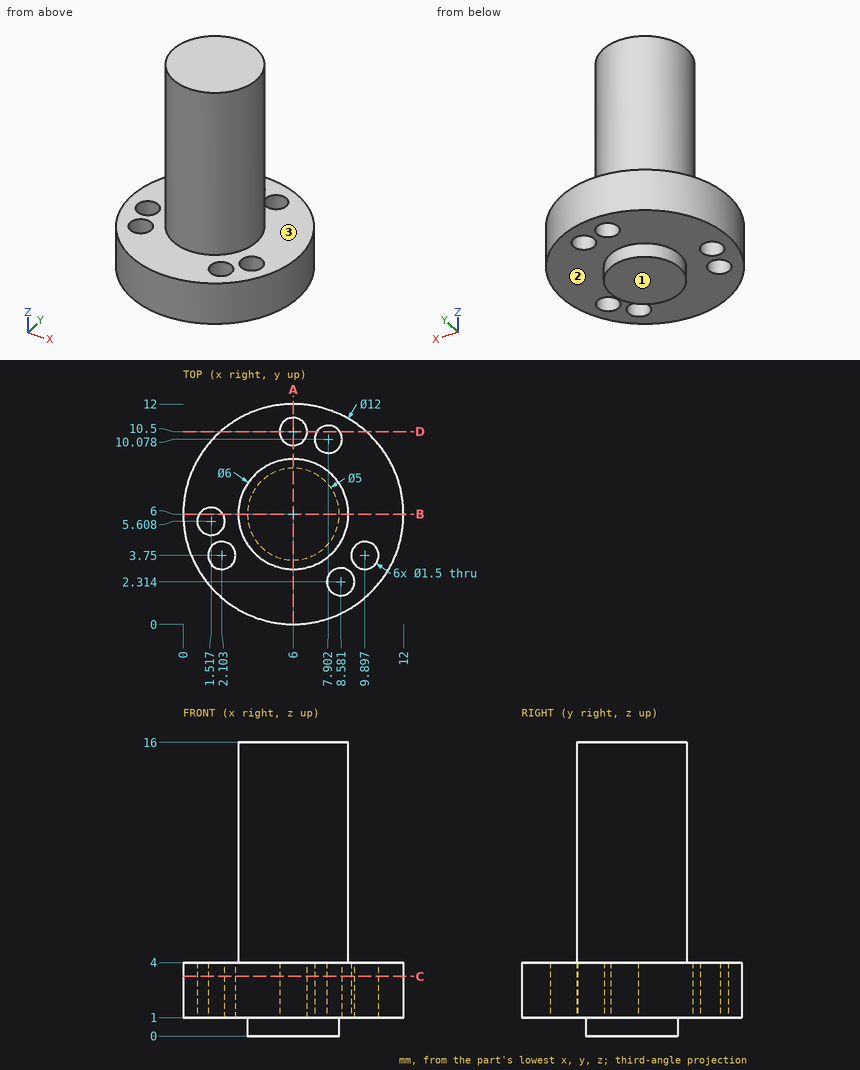
Design review of the part shown in the three views and the two pictorial views. Dimensions are in mm from the part's minimum x, y and z. A direction names the side the tool comes from. Round coordinates to 2 decimals unless told otherwise and drop trailing zeros. Order: outer loops, then holes, each group sorted by start corner. A loop starts at its lowest first (then second) coordinate and runs counter-clockwise, first axis right, second up.
Q1. Wall thickness on line 1 (Y direction, x = 6, z = 2.15); line 2 (Y direction, x = 8.25, z = 2.5) (1 decimal); line 3 (Z direction, x = 3.5, y = 8.25): over which ranges is each line inside the solid? List them lowest first.
Findings below:
line 1: y = 0 to 9.75, 11.25 to 12
line 2: y = 0.4 to 1.6, 3 to 9.4, 10.7 to 11.6
line 3: z = 1 to 4
Q2. We need section A-A, the plane x = 6. Give the boundary of the cut face in (y, z), plus the area to 4 significant figures.
Findings below:
outline: (0, 1) - (3.5, 1) - (3.5, 0) - (8.5, 0) - (8.5, 1) - (9.75, 1) - (9.75, 4) - (9, 4) - (9, 16) - (3, 16) - (3, 4) - (0, 4) - close; (11.25, 1) - (12, 1) - (12, 4) - (11.25, 4) - close
area: 108.5 mm2
Q3. Machinability: for the marked faces 1, 2 and 3, which of the approach directions +Z, -Z, +X, -X, +Y, -Y give a long, thin tool a straight path to every point of the face, cutting with its end or side? Answer none if there is none.
Findings below:
face 1: -Z, +X, -X, +Y, -Y
face 2: -Z
face 3: +Z
Q4. Insertion check: P1, Ø2, axis at x = 7.9, y = 10.08, coming from the +Z side; P2, Ø0.9, axis at x = 9.9, y = 3.75, coming from the -Z side; P3, Ø2, axis at y = 4.5, z = 2.5, coming from the +X side; P4, Ø3, axis at x = 8, y = 6, coming from the -Z side. Each pin has a flat end and moves straight along its axis. Give the tip position at first contact, or say it passes through.
Findings below:
P1: stops at z = 4
P2: passes through
P3: stops at x = 11.98
P4: stops at z = 0
Q5. We need section B-B, the plane y = 6. Give the boundary of the cut face in (x, z), plus the area to 3 significant figures.
Findings below:
outline: (0, 1) - (0.88, 1) - (0.88, 4) - (0, 4) - close; (2.16, 1) - (3.5, 1) - (3.5, 0) - (8.5, 0) - (8.5, 1) - (12, 1) - (12, 4) - (9, 4) - (9, 16) - (3, 16) - (3, 4) - (2.16, 4) - close
area: 109 mm2
Q6. We need section D-D, the plane y = 10.5. Give the boundary of the cut face in (x, z).
Findings below:
outline: (2.03, 1) - (5.25, 1) - (5.25, 4) - (2.03, 4) - close; (6.75, 1) - (7.28, 1) - (7.28, 4) - (6.75, 4) - close; (8.52, 1) - (9.97, 1) - (9.97, 4) - (8.52, 4) - close
Q7. We need section C-C, the plane z = 3.25. Give the boundary of the cut face in (x, y).
Findings below:
outline: circle Ø12 at (6, 6); hole circle Ø1.5 at (1.52, 5.61); hole circle Ø1.5 at (2.1, 3.75); hole circle Ø1.5 at (6, 10.5); hole circle Ø1.5 at (7.9, 10.08); hole circle Ø1.5 at (8.58, 2.31); hole circle Ø1.5 at (9.9, 3.75)
